Here's the drawing with two shaded views (mm, measured from the low corner). I have some questions. Coordinates: 2 decimals unless noted, no trailing zeros. Loops run counter-clockwise (first coordinate to the right, second up) from the corner with the lowest first, then second, coordinate; pieces in that order, holes last. Notation, with made-up numbers: (52, -26.75) - (90, -26.75) arc R12 ccw to (90, -14.75) - close; hole circle Ø4 at (74, 32). An arc over 180 degrees is marked (long way). Use a Markdown table: item, result.
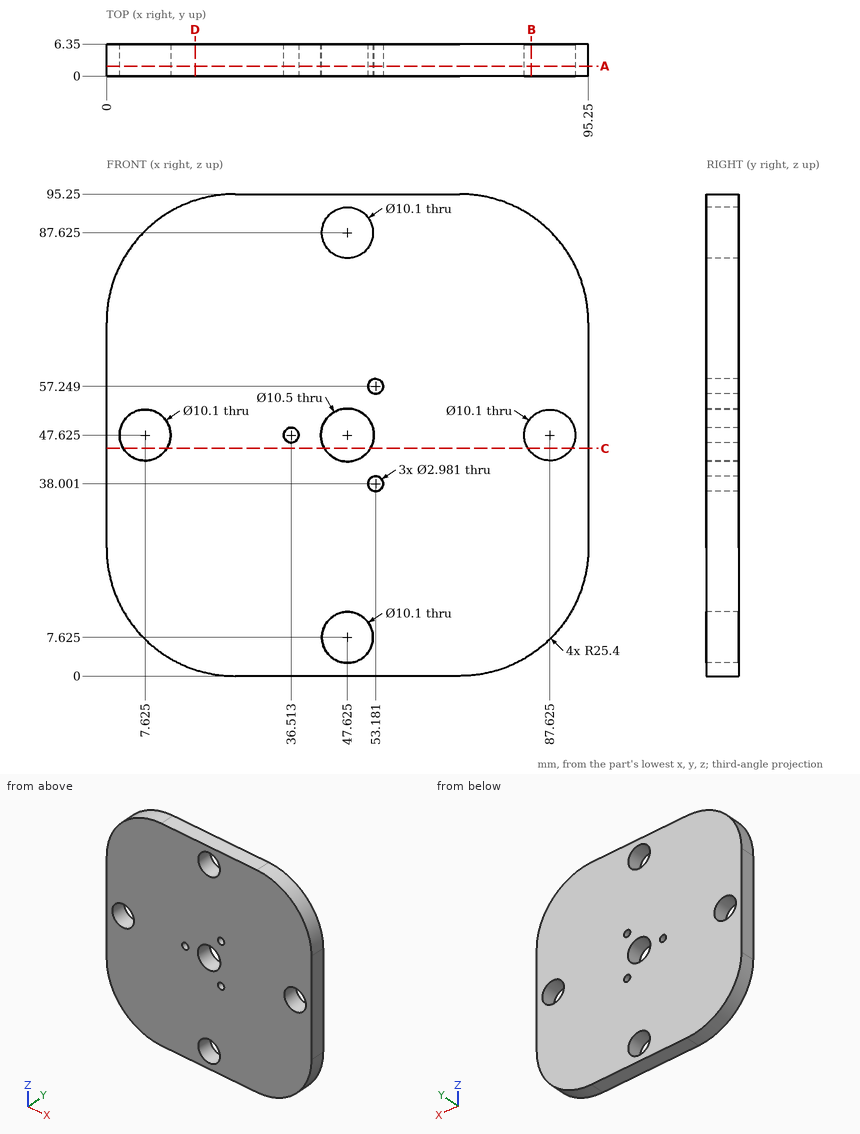
Q1. I want a section at A-A, the plane y = 2. Give the number of separate pieces and of enclosed holes in the cut face, then the cut area to 3 significant figures.
Check values:
| item | result |
|---|---|
| separate pieces | 1 |
| enclosed holes | 8 |
| area | 8,090 mm^2 |
Q2. Will these pins go through, and if not, where does the flat tip stop? P1, Ø2.5, axis at x = 36.51, z = 47.62, coming from the -Y side; P2, Ø1, axis at y = 1, z = 49.5, coming from the -X side; P3, Ø3, axis at y = 5, z = 78.5, coming from the +X side.
Check values:
| item | result |
|---|---|
| P1 | through |
| P2 | x = 0 |
| P3 | x = 94.22 |
Q3. I want a section at C-C, the plane z = 45. Write out the boundary of the cut face in (x, y).
Check values:
| item | result |
|---|---|
| outline | (0, 0) - (3.31, 0) - (3.31, 6.35) - (0, 6.35) - close; (11.94, 0) - (43.08, 0) - (43.08, 6.35) - (11.94, 6.35) - close; (52.17, 0) - (83.31, 0) - (83.31, 6.35) - (52.17, 6.35) - close; (91.94, 0) - (95.25, 0) - (95.25, 6.35) - (91.94, 6.35) - close |
Q4. Please list where these lines run through material, in increasing order: L1, parallel to Z at x = 53, y = 5.75; L2, parallel to X at y = 2.5, z = 38; L3, parallel to Z at x = 45, y = 4.5. Write a range as from..to.
Check values:
| item | result |
|---|---|
| L1 | 0..36.52, 39.48..55.77, 58.73..95.25 |
| L2 | 0..51.69, 54.67..95.25 |
| L3 | 0..3.31, 11.94..43.08, 52.17..83.31, 91.94..95.25 |
Q5. I want a section at D-D, the plane x = 17.5. Write out the boundary of the cut face in (y, z), then the cut area to 3 significant figures.
Check values:
| item | result |
|---|---|
| outline | (0, 1.26) - (6.35, 1.26) - (6.35, 93.99) - (0, 93.99) - close |
| area | 589 mm^2 |
Q6. I want a section at B-B, the plane x = 84. Write out the boundary of the cut face in (y, z).
Check values:
| item | result |
|---|---|
| outline | (0, 4.31) - (6.35, 4.31) - (6.35, 44.11) - (0, 44.11) - close; (0, 51.14) - (6.35, 51.14) - (6.35, 90.94) - (0, 90.94) - close |
